```python
from build123d import *

# Parameters (mm, degrees)
CUT_EXTRUDE2_DEPTH      = 3112.786644088
CUT_EXTRUDE2_DEPTH_BACK = 3112.786644088
SKETCH2_OUTSIDE_W       = 3550.624
SKETCH2_OUTSIDE_H       = 1823.424
SKETCH2_OUTSIDE_W_2     = 184.404
SKETCH2_OUTSIDE_H_2     = 50.292
CUT_EXTRUDE3_START      = 6.35
SKETCH3_W               = 184.404
SKETCH3_H               = 50.292
CUT_EXTRUDE3_DEPTH      = 2742.052714982
SKETCH4_R               = 3.429
CUT_EXTRUDE4_DEPTH      = 96.78023097


with BuildPart() as part:
    # Sketch1 → Revolve1 (revolve)
    with BuildSketch(Plane.XY):
        with BuildLine():
            Line((1372.87, -509.27), (1372.87, 509.27))
            add(Edge.make_bspline(
                [(1372.87, 509.27), (0, 509.27), (0, 0), (0, -509.27), (1372.87, -509.27)],
                knots=[4.71238898, 4.71238898, 4.71238898, 6.283185307, 6.283185307, 7.853981634, 7.853981634, 7.853981634], degree=2, weights=[1, 0.707106781, 1, 0.707106781, 1]))
        make_face()
    revolve(axis=Axis((1372.87, -509.27, 0), (0, 1, 0)))

    # Sketch2 outside → Cut-Extrude2 (cut, two sides: drawn at the far end of the back side and taken through both)
    with BuildSketch(Plane(origin=(0, 0, 0), x_dir=(0, 0, -1), z_dir=(1, 0, 0)).offset(-CUT_EXTRUDE2_DEPTH_BACK)):
        Rectangle(SKETCH2_OUTSIDE_W, SKETCH2_OUTSIDE_H)
        Rectangle(SKETCH2_OUTSIDE_W_2, SKETCH2_OUTSIDE_H_2, mode=Mode.SUBTRACT)
    extrude(amount=CUT_EXTRUDE2_DEPTH + CUT_EXTRUDE2_DEPTH_BACK, mode=Mode.SUBTRACT)

    # Sketch3 → Cut-Extrude3 (cut, through all)
    with BuildSketch(Plane(origin=(0, 0, 0), x_dir=(0, 0, -1), z_dir=(1, 0, 0)).offset(CUT_EXTRUDE3_START)):
        Rectangle(SKETCH3_W, SKETCH3_H)
    extrude(amount=CUT_EXTRUDE3_DEPTH, mode=Mode.SUBTRACT)

    # Sketch4 → Cut-Extrude4 (cut, through all)
    with BuildSketch(Plane(origin=(6.35, 0, 0), x_dir=(0, 0, -1), z_dir=(1, 0, 0))):
        with Locations((-85.852, 18.796)):
            Circle(SKETCH4_R)
        with Locations((-85.852, -18.796)):
            Circle(SKETCH4_R)
        with Locations((85.852, -18.796)):
            Circle(SKETCH4_R)
        with Locations((85.852, 18.796)):
            Circle(SKETCH4_R)
    extrude(amount=-CUT_EXTRUDE4_DEPTH, mode=Mode.SUBTRACT)


solid = part.part
```
Verification items for the finished model (mm, model axes). Round coordinates to 2 decimals unless told otherwise and drop trailing zeros. Write each question's results on one line, items separated by ' | '.
Q1. Go/stop test with flat-tipped pins: pin 1 Ø11 at (y, z) = (-18.796, 85.852) entering from +X; pin 2 Ø6 at (y, z) = (-18.796, -85.852) entering from +X. Record where each tip stops, or that it passes through.
Derived:
pin 1: stops at x = 6.35 | pin 2: passes through
Q2. Thickness scan on probe 1 along Z at (x, y) = (5.5, 21); probe 2 along X at (y, z) = (-3, 62); probe 3 along X at (y, z) = (12.5, 63.5). Record the ranges inside material, lowest first.
Derived:
probe 1: z = -92.2 to -88.48, -83.23 to 83.23, 88.48 to 92.2 | probe 2: x = 1.42 to 6.35 | probe 3: x = 1.88 to 6.35
Q3. Sectioned sample at A-A, the plane y = 20.5. Give the number of separate pieces and of enclosed holes in the cut face, and give its area (3 significant figures).
Derived:
separate pieces: 3 | enclosed holes: 0 | area: 745 mm²
Q4. Draft check along Z on faces 1 (the face through (4, 25.146, 1)), 2 (the face through (5, 0, 92.202)), 3 (the face through (4.818, -16.479, -83.325)). Enter one of: released by +Z, released by -Z, zero draft, split by the parting line, or undercut.
Derived:
face 1: zero draft | face 2: released by +Z | face 3: undercut
